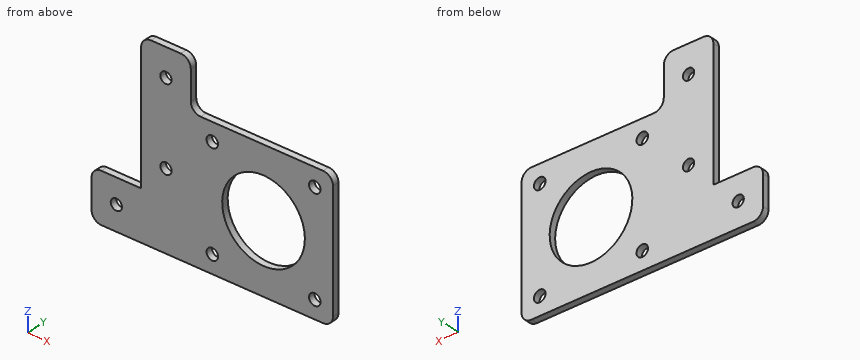
```python
from build123d import *

# Parameters (mm, degrees)
SKETCH_1_R      = 12.5
SKETCH_1_R_2    = 1.75
SKETCH_1_R_3    = 1.7
EXTRUDE_2_DEPTH = 2


with BuildPart() as part:
    # 草图1 → 凸台-拉伸2 (new body)
    with BuildSketch(Plane(origin=(0, 0, 0), x_dir=(1, 0, 0), z_dir=(0, 1, 0))):
        with BuildLine():
            Line((0, 0), (-12, 0))
            ThreePointArc((-12, 0), (-14.121320344, 0.878679656), (-15, 3))
            Line((-15, 3), (-15, 12))
            ThreePointArc((-15, 12), (-14.121320344, 14.121320344), (-12, 15))
            Line((-12, 15), (15, 15))
            Line((15, 15), (55, 15))
            ThreePointArc((55, 15), (57.121320344, 14.121320344), (58, 12))
            Line((58, 12), (58, -24))
            ThreePointArc((58, -24), (57.121320344, -26.121320344), (55, -27))
            Line((55, -27), (18, -27))
            ThreePointArc((18, -27), (15.878679656, -27.878679656), (15, -30))
            Line((15, -30), (15, -39))
            ThreePointArc((15, -39), (14.121320344, -41.121320344), (12, -42))
            Line((12, -42), (3, -42))
            ThreePointArc((3, -42), (0.878679656, -41.121320344), (0, -39))
            Line((0, -39), (0, -32.824659397))
            Line((0, -32.824659397), (0, 0))
        make_face()
        with Locations(Location((37, -6, 0), (0, 0, 270))):
            Circle(SKETCH_1_R, mode=Mode.SUBTRACT)
        with Locations(Location((52.5, -21.5, 0), (0, 0, 270))):
            Circle(SKETCH_1_R_2, mode=Mode.SUBTRACT)
        with Locations(Location((21.5, -21.5, 0), (0, 0, 270))):
            Circle(SKETCH_1_R_2, mode=Mode.SUBTRACT)
        with Locations(Location((21.5, 9.5, 0), (0, 0, 90))):
            Circle(SKETCH_1_R_2, mode=Mode.SUBTRACT)
        with Locations(Location((52.5, 9.5, 0), (0, 0, 90))):
            Circle(SKETCH_1_R_2, mode=Mode.SUBTRACT)
        with Locations(Location((7.5, -8.5, 0), (0, 0, 270))):
            Circle(SKETCH_1_R_3, mode=Mode.SUBTRACT)
        with Locations(Location((7.5, -33.5, 0), (0, 0, 270))):
            Circle(SKETCH_1_R_3, mode=Mode.SUBTRACT)
        with Locations(Location((-7.5, 7.5, 0), (0, 0, 270))):
            Circle(SKETCH_1_R_3, mode=Mode.SUBTRACT)
    extrude(amount=EXTRUDE_2_DEPTH)


solid = part.part
```
Input: part model. Units: mm. Frame: model coordinates. Round coordinates to 2 decimals unless told otherwise and drop trailing zeros. Order: outer loops, then holes, each group sorted by start corner. A loop starts at its lowest first (then second) coordinate and runs counter-clockwise, first axis right, second up. Notation, with made-up numbers: (76, 40) - (118, 40) arc R20 ccw to (118, 75) - close; hole circle Ø9 at (-11.5, -15). An arc over 180 degrees is marked (long way). One line per question, with ' | ' between items. Start each with the question number.
1) Cut plane A-A, the plane z = 16. Return the cut outline in (x, y).
2) Contact query for flat-ended pins moving along their axis: P1, Ø1.5, axis at x = 10, z = 11, coming from the -Y side; P2, Ø1, axis at x = 18, y = 0.5, coming from the +Z side; P3, Ø3, axis at x = 52.5, z = -9.5, coming from the +Y side; P4, Ø0.6, axis at y = 1, z = 24, coming from the -X side. Output: stop coordinate, or through.
3) Cut plane C-C, the plane y = 0.5. Give the number of separate pieces and of enclosed holes in the cut face, then the cut area to 3 significant figures.
4) Cut plane B-B, the plane x = 21.5. Return the cut outline in (y, z), then the cut area to 3 significant figures.
5) Cut plane D-D, the plane z = 33.5. Return the cut outline in (x, y).
6) Ray query, probe 1 along X at (y, z) = (1, 21.5); probe 2 along X at (y, z) = (1.55, -9.5); probe 3 along X at (y, z) = (0.7, 6). Return the intervals inside material, ascending.
Worked out:
1) outline: (0, 0) - (29.5, 0) - (29.5, 2) - (0, 2) - close; (44.5, 0) - (58, 0) - (58, 2) - (44.5, 2) - close
2) P1: stops at y = 0 | P2: stops at z = 27.04 | P3: passes through | P4: stops at x = 0
3) separate pieces: 1 | enclosed holes: 8 | area: 2,320 mm^2
4) outline: (0, -15) - (2, -15) - (2, -11.25) - (0, -11.25) - close; (0, -7.75) - (2, -7.75) - (2, 19.75) - (0, 19.75) - close; (0, 23.25) - (2, 23.25) - (2, 27) - (0, 27) - close | area: 70.0 mm^2
5) outline: (0, 0) - (5.8, 0) - (5.8, 2) - (0, 2) - close; (9.2, 0) - (15, 0) - (15, 2) - (9.2, 2) - close
6) probe 1: x = 0 to 19.75, 23.25 to 50.75, 54.25 to 58 | probe 2: x = -15 to 19.75, 23.25 to 50.75, 54.25 to 58 | probe 3: x = 0 to 24.5, 49.5 to 58
